Part print with two shaded views. Sizes in mm from the minimum x, y, z corner. A direction names the side the tool comes from. Round coordinates to 2 decimals unless told otherwise and drop trailing zeros. Loops run counter-clockwise (first coordinate to the right, second up) from the corner with the lowest first, then second, coordinate; pieces in that order, holes last. Notation, with made-up numbers: (63, 50.5) - (78, 50.5) arc R20 ccw to (78, 88.5) - close; hole circle Ø1 at (-31, 65.25). An arc over 180 degrees is marked (long way). Use a Markdown table: item, result.
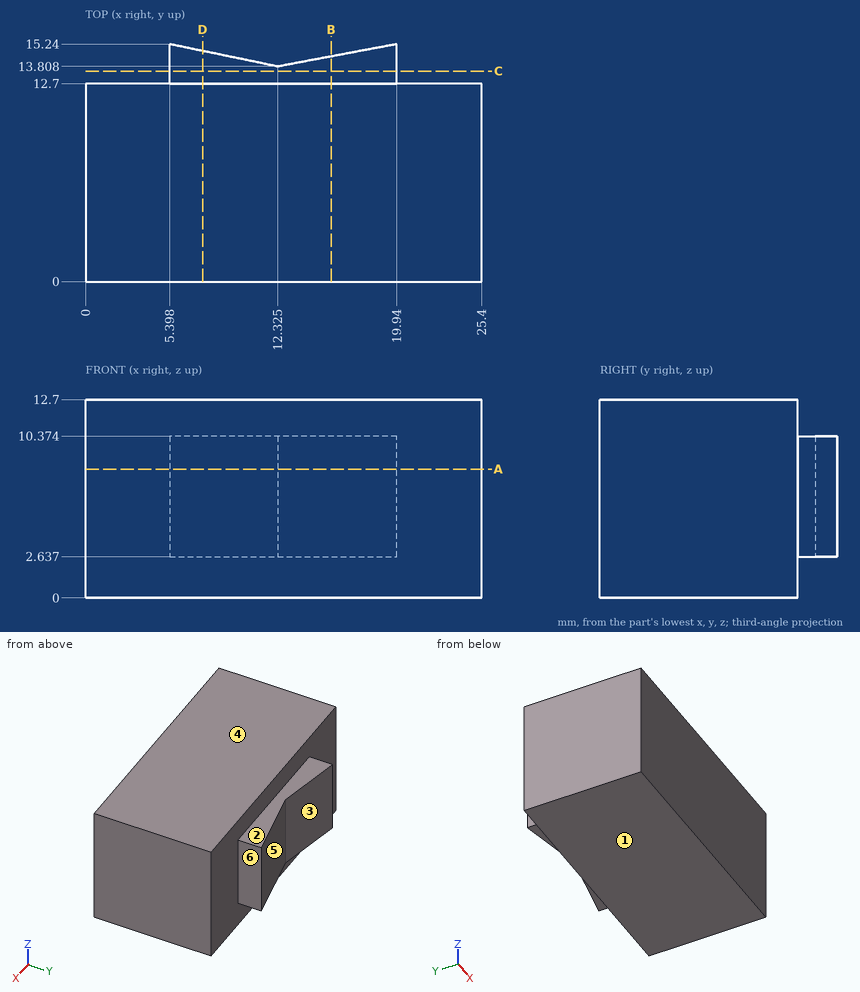
Q1. Cut at D-D, the plane x = 7.5. List the corners of the cut face in (y, z).
Results found:
| item | result |
|---|---|
| outline | (0, 0) - (12.7, 0) - (12.7, 2.64) - (14.81, 2.64) - (14.81, 10.37) - (12.7, 10.37) - (12.7, 12.7) - (0, 12.7) - close |
Q2. Cut at C-C, the plane y = 13.5. List the corners of the cut face in (x, z).
Results found:
| item | result |
|---|---|
| outline | (5.4, 2.64) - (19.94, 2.64) - (19.94, 10.37) - (5.4, 10.37) - close |
Q3. Which spindle directions (+Z, -Z, +X, -X, +Y, -Y) get a long thin tool onto all of the face, cutting with end or side? Do the marked faces 1 and 2. Say none if no direction does.
Results found:
| item | result |
|---|---|
| face 1 | -Z, +X, -X, +Y, -Y |
| face 2 | +Z, +X, -X, +Y |
Q4. Pull direction X, two halves, no side cores. Call the marked faces 3, 4, 5 and 6: pulls with the +X half, pulls with the -X half, needs draft (parallel to the pull), parting line crosses it, or undercut.
Results found:
| item | result |
|---|---|
| face 3 | undercut |
| face 4 | needs draft |
| face 5 | undercut |
| face 6 | pulls with the +X half |
Q5. Probe line 1 (X direction, y = 13, z = 8); line 2 (Z direction, x = 14, y = 14); line 3 (Y direction, x = 20.75, z = 10.25). List the from-to ranges inside material, lowest first.
Results found:
| item | result |
|---|---|
| line 1 | x = 5.4 to 19.94 |
| line 2 | z = 2.64 to 10.37 |
| line 3 | y = 0 to 12.7 |
Q6. Drop flat-ended pins along their axis: pin 1 (0.8 mm diameter, centred on x = 9, y = 13.5, fed in from +Z); pin 2 (4 mm diameter, centred on x = 14.5, z = 3.5, fed in from +Y); pin 3 (2 mm diameter, centred on x = 3.5, z = 7, fed in from +Y). Give the stop position or say it passes through.
Results found:
| item | result |
|---|---|
| pin 1 | stops at z = 10.37 |
| pin 2 | stops at y = 14.59 |
| pin 3 | stops at y = 12.7 |
Q7. Cut at B-B, the plane x = 15.75. List the corners of the cut face in (y, z).
Results found:
| item | result |
|---|---|
| outline | (0, 0) - (12.7, 0) - (12.7, 2.64) - (14.45, 2.64) - (14.45, 10.37) - (12.7, 10.37) - (12.7, 12.7) - (0, 12.7) - close |
Q8. Cut at A-A, the plane z = 8.25. List the corners of the cut face in (x, y) (1 decimal), plus the area to 3 significant figures.
Results found:
| item | result |
|---|---|
| outline | (0, 0) - (25.4, 0) - (25.4, 12.7) - (19.9, 12.7) - (19.9, 15.2) - (12.3, 13.8) - (5.4, 15.2) - (5.4, 12.7) - (0, 12.7) - close |
| area | 349 mm2 |
